from build123d import *

# Parameters (mm, degrees)
CUT_THICKEN1_START             = -161.779064873
CUT_THICKEN1_DEPTH             = 1.271941736
F_3_0_3_DIAMETER_HOLE1_D       = 3
F_3_0_3_DIAMETER_HOLE1_DEPTH   = 6.997347225
F_2_5_2_5_DIAMETER_HOLE1_D     = 2.5
F_2_5_2_5_DIAMETER_HOLE1_DEPTH = 60.082245303
F_2_5_2_5_DIAMETER_HOLE2_D     = 2.5
F_2_5_2_5_DIAMETER_HOLE2_DEPTH = 338.689419568


# Read off the part's stored shape, not the designer's step: Cut-Thicken1
with BuildPart() as part:
    # Sketch1 → Revolve1 (revolve)
    with BuildSketch(Plane(origin=(-300, 0, 0), x_dir=(0, -1, 0), z_dir=(-1, 0, 0)), mode=Mode.PRIVATE) as revolve1_sk:
        with BuildLine():
            Line((-527.332012287, -352.357743681), (-528.839135448, -364.91710336))
            Line((-528.839135448, -364.91710336), (-528.839135448, -377.357743681))
            Line((-528.839135448, -377.357743681), (-527.839135448, -377.357743681))
            Line((-527.839135448, -377.357743681), (-527.839135448, -364.976888902))
            Line((-527.839135448, -364.976888902), (-526.339135448, -352.476888902))
            ThreePointArc((-526.339135448, -352.476888902), (-525.203611847, -349.572885006), (-522.332012286, -348.357743681))
            ThreePointArc((-522.332012286, -348.357743681), (-521.849911622, -347.857743681), (-522.332012286, -347.357743681))
            ThreePointArc((-522.332012286, -347.357743681), (-525.867546192, -348.822209775), (-527.332012287, -352.357743681))
        make_face()
    revolve(revolve1_sk.sketch.rotate(Axis((-300, 667.332012286, -347.075887645), (0, 0, -1)), 90), axis=Axis((-300, 667.332012286, -347.075887645), (0, 0, -1)))

    # Cut-Thicken1 outline → Cut-Thicken1 (cut)
    with BuildSketch(Plane.YZ.offset(CUT_THICKEN1_START)):
        with BuildLine():
            ThreePointArc((676.006688073, -377.357743681), (667.332012287, -373.857743681), (658.6573365, -377.357743681))
            Line((658.6573365, -377.357743681), (676.006688073, -377.357743681))
        make_face()
    extrude(amount=CUT_THICKEN1_DEPTH, mode=Mode.SUBTRACT)

    # Ø3.0 (3) Diameter Hole1
    with Locations(Plane.ZY.offset(161.515246561)):
        with Locations((-369.357743681, 667.332012286)):
            Hole(F_3_0_3_DIAMETER_HOLE1_D / 2, depth=F_3_0_3_DIAMETER_HOLE1_DEPTH)

    # Ø2.5 (2.5) Diameter Hole1
    with Locations(Plane(origin=(-294.638237699, 510.328397547, 0), x_dir=(0.866025403784442, 0.4999999999999941, 0), z_dir=(-0.49999999999999417, 0.8660254037844421, 0))):
        with Locations((73.858385008, 362.357743681)):
            Hole(F_2_5_2_5_DIAMETER_HOLE1_D / 2, depth=F_2_5_2_5_DIAMETER_HOLE1_DEPTH)

    # Ø2.5 (2.5) Diameter Hole2
    with Locations(Plane(origin=(283.941824832, 491.801667003, 0), x_dir=(0.8660254037844352, -0.5000000000000062, 0), z_dir=(0.5000000000000061, 0.866025403784435, 0))):
        with Locations((-593.473627278, 362.357743681)):
            Hole(F_2_5_2_5_DIAMETER_HOLE2_D / 2, depth=F_2_5_2_5_DIAMETER_HOLE2_DEPTH)


solid = part.part
The model under review builds one solid part; all positions refer to its coordinate system, in mm. A direction names the side the tool comes from. Round coordinates to 2 decimals unless told otherwise and drop trailing zeros. One line per item, written item: value. Start each with the question number.
1. Machinability: for faces 1 (the face through (-190.039, 583.017, -364.307)), 2 (the face through (-428.86, 613.91, -371.08)), which of the approach directions +Z, -Z, +X, -X, +Y, -Y give a long, thin tool a straight path to every point of the face, cutting with its end or side? Answer none if there is none.
2. The part is to be moulded in two halves that separate along Y. For faces 3 (the face through (-432.1, 708.93, -371.22)), 4 (the face through (-269.74, 531.065, -364.195)), say which applies: released by +Y, released by -Y, zero draft, split by the parting line, or undercut.
3. Clearance check with flat-ended pins moving along their axes: P1, Ø2, axis at x = -214.5, z = -362, coming from the -Y side; P2, Ø5, axis at y = 765.5, z = -353, coming from the -X side; P3, Ø1.5, axis at x = -360.5, z = -360.5, coming from the +Y side. State where each tip first meets the part, or that it passes through.
4. To check wall thickness, follow L1, parallel to X at y = 665.5, z = -368; L2, parallel to Y at x = -300, z = -371; L3, parallel to Y at x = -305.5, z = -364. State the ranges of each line that lie inside material, in increasing order. Write a range as from..to.
Checks:
1. face 1: +Z
1. face 2: -Z
2. face 3: undercut
2. face 4: split by the parting line
3. P1: stops at y = 555.88
3. P2: stops at x = -403.52
3. P3: stops at y = 793.99
4. L1: x = -439.48..-438.48, -161.52..-160.52
4. L2: y = 527.84..528.84, 805.82..806.82
4. L3: y = 527.83..528.84, 805.83..806.83
